For this review, take the finished solid that the model builds, in its own axes (mm). Face numbers are marked on the shaded views. A direction names the side the tool comes from. Round coordinates to 2 decimals unless told otherwise and drop trailing zeros. Write each loop counter-clockwise with the first axis right and the second up, starting at its lowest first coordinate (ties: lowest second). Pieces come first, ordered by that corner, then holes. Notation, with made-up numbers: M 73,-26.5 L 112,-26.5 A14 cw 112,-4.5 Z; hole C 25,-23.75 d2. An arc over 180 degrees is marked long. One line per question, with ' | ' between items.
```python
from build123d import *

# Parameters (mm, degrees)
ESQUISSE1_R             = 2.75
BOSS_EXTRU_1_DEPTH      = 2.5
ESQUISSE2_R             = 1.5
BOSS_EXTRU_2_DEPTH      = 10
ESQUISSE3_W             = 7.386684128
ESQUISSE3_H             = 0.735038592
ENL_V_MAT_EXTRU_1_DEPTH = 0.75


with BuildPart() as part:
    # Esquisse1 → Boss.-Extru.1 (new body)
    with BuildSketch(Plane.XY):
        Circle(ESQUISSE1_R)
    extrude(amount=BOSS_EXTRU_1_DEPTH)

    # Esquisse2 → Boss.-Extru.2 (add)
    with BuildSketch(Plane.XY.offset(2.5)):
        Circle(ESQUISSE2_R)
    extrude(amount=BOSS_EXTRU_2_DEPTH)

    # Esquisse3 → Enlèv. mat.-Extru.1 (cut)
    with BuildSketch(Plane(origin=(0, 0, 0), x_dir=(-1, 0, 0), z_dir=(0, 0, -1))):
        Rectangle(ESQUISSE3_W, ESQUISSE3_H)
    extrude(amount=-ENL_V_MAT_EXTRU_1_DEPTH, mode=Mode.SUBTRACT)


solid = part.part
```
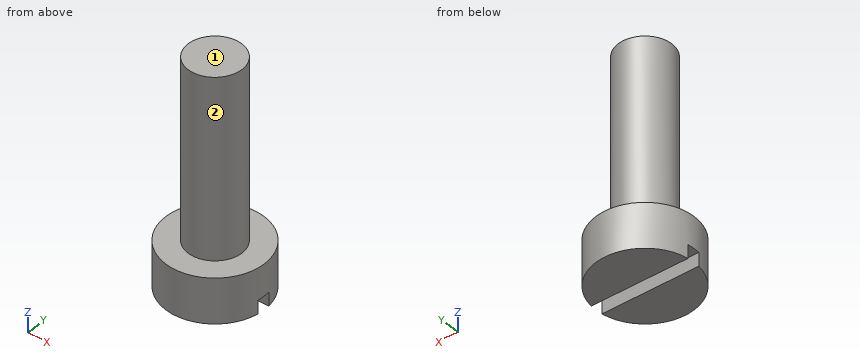
Item 1: Insertion check: pin 1 Ø2 at (x, z) = (-2, 4.5) entering from -Y; pin 2 Ø2 at (x, z) = (0.5, 9.5) entering from -Y; pin 3 Ø1.5 at (y, z) = (-0.5, 4) entering from -X. Each pin has a flat end and moves straight along its axis. Give the tip position at first contact, or say it passes through.
Results:
pin 1: y = -1.12 | pin 2: y = -1.5 | pin 3: x = -1.5
Item 2: Machinability: for the marked faces 1 and 2, which of the approach directions +Z, -Z, +X, -X, +Y, -Y give a long, thin tool a straight path to every point of the face, cutting with its end or side? Answer none if there is none.
Results:
face 1: +Z, +X, -X, +Y, -Y | face 2: +Z
Item 3: Take a section at D-D (x = -0.9). Write out the cut boundary in (y, z), then the cut area to 3 significant figures.
Results:
outline: M -2.6,0 L -0.37,0 L -0.37,0.75 L 0.37,0.75 L 0.37,0 L 2.6,0 L 2.6,2.5 L 1.2,2.5 L 1.2,12.5 L -1.2,12.5 L -1.2,2.5 L -2.6,2.5 Z | area: 36.4 mm2
Item 4: Take a section at B-B (x = 0). Write out the cut boundary in (y, z).
Results:
outline: M -2.75,0 L -0.37,0 L -0.37,0.75 L 0.37,0.75 L 0.37,0 L 2.75,0 L 2.75,2.5 L 1.5,2.5 L 1.5,12.5 L -1.5,12.5 L -1.5,2.5 L -2.75,2.5 Z
Item 5: Take a section at A-A (y = 0). Write out the cut boundary in (x, z), then the cut area to 3 significant figures.
Results:
outline: M -2.75,0.75 L 2.75,0.75 L 2.75,2.5 L 1.5,2.5 L 1.5,12.5 L -1.5,12.5 L -1.5,2.5 L -2.75,2.5 Z | area: 39.6 mm2
Item 6: Take a section at C-C (z = 6.5). Write out the cut boundary in (x, y).
Results:
outline: C 0,0 d3
Item 7: To check wall thickness, follow line 1 along Y through (x, z) = (0.05, 4.25); line 2 along Z through (x, y) = (1.85, -1.4); line 3 along Z through (x, y) = (0.4, 0.05). State the ranges of each line that lie inside material, in increasing order. Write a range as from..to.
Results:
line 1: -1.5..1.5 | line 2: 0..2.5 | line 3: 0.75..12.5
